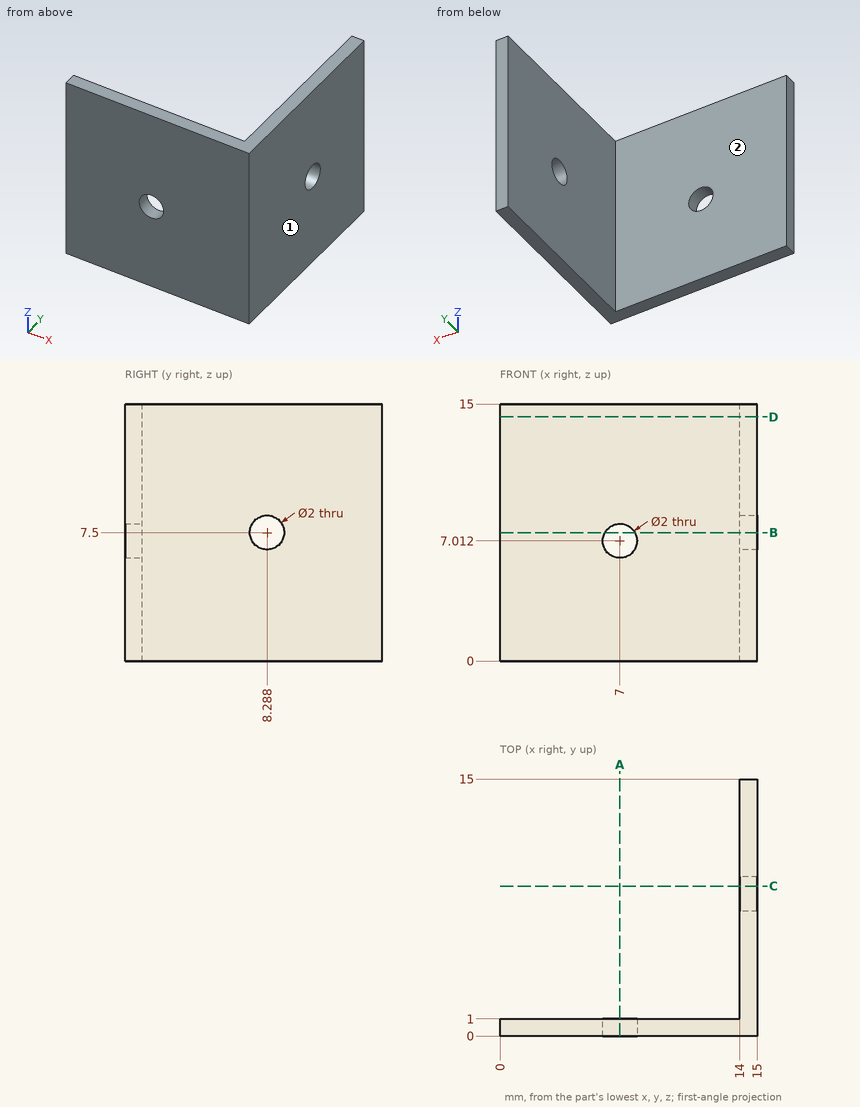
Input: dimensioned drawing with shaded views. Units: mm. Origin: part minimum x, y, z. A direction names the side the tool comes from. Give positions to 0.01 mm unless a question says otherwise; leave off trailing zeros. Order: outer loops, then holes, each group sorted by start corner. A loop starts at its lowest first (then second) coordinate and runs counter-clockwise, first axis right, second up. Notation, with made-up numbers: (54.5, 57.25) -> (66.5, 57.25) arc R18 cw to (66.5, 62.25) -> close; hole circle Ø2 at (5.25, 40). An arc over 180 degrees is marked (long way). Answer as a JSON object with one key per item and string values.
Q1. Section D-D (z = 14.25). Output: boundary loops of the cut face in (x, y), plus the area to 3 significant figures.
Entries:
{"outline": "(0, 0) -> (15, 0) -> (15, 15) -> (14, 15) -> (14, 1) -> (0, 1) -> close", "area": "29.0 mm^2"}
Q2. Material intervals for probe 1 along Y at (x, z) = (14.7, 7.5); probe 2 along Z at (x, y) = (7, 0.5); probe 3 along Y at (x, z) = (1, 3.5), sorted ascending.
Entries:
{"probe 1": "y = 0 to 7.29, 9.29 to 15", "probe 2": "z = 0 to 6.01, 8.01 to 15", "probe 3": "y = 0 to 1"}
Q3. First-contact query: pin 1 (4 mm diameter, centred on x = 5.5, z = 10, fed in from +Y); pin 2 (3 mm diameter, centred on y = 8.29, z = 7.5, fed in from -X); pin 3 (1.8 mm diameter, centred on x = 7, z = 7.01, fed in from +Y). Flat tips, straight axial feed; report the tip coordinate or a pass-through.
Entries:
{"pin 1": "stops at y = 1", "pin 2": "stops at x = 14", "pin 3": "passes through"}
Q4. Access query for the marked faces 1 and 2. Directions: +Z, -Z, +X, -X, +Y, -Y. A direction counts if a zero-diameter tool reaches every point of the face in a straight line with its end or side. Return the directions, or none.
Entries:
{"face 1": "+Z, -Z, +X, +Y, -Y", "face 2": "+Z, -Z, -X, +Y"}
Q5. Section C-C (y = 8.75). Output: boundary loops of the cut face in (x, z).
Entries:
{"outline": "(14, 0) -> (15, 0) -> (15, 6.61) -> (14, 6.61) -> close; (14, 8.39) -> (15, 8.39) -> (15, 15) -> (14, 15) -> close"}
Q6. Section B-B (z = 7.5). Output: boundary loops of the cut face in (x, y).
Entries:
{"outline": "(0, 0) -> (6.13, 0) -> (6.13, 1) -> (0, 1) -> close; (7.87, 0) -> (15, 0) -> (15, 7.29) -> (14, 7.29) -> (14, 1) -> (7.87, 1) -> close; (14, 9.29) -> (15, 9.29) -> (15, 15) -> (14, 15) -> close"}
Q7. Section A-A (x = 7). Output: boundary loops of the cut face in (y, z), plus the area to 3 significant figures.
Entries:
{"outline": "(0, 0) -> (1, 0) -> (1, 6.01) -> (0, 6.01) -> close; (0, 8.01) -> (1, 8.01) -> (1, 15) -> (0, 15) -> close", "area": "13.0 mm^2"}
